Design review of the part built by this model. Coordinates are the model's own, in mm. Round coordinates to 2 decimals unless told otherwise and drop trailing zeros. Write each loop counter-clockwise with the first axis right and the second up, starting at its lowest first coordinate (ties: lowest second). Pieces come first, ordered by that corner, then holes. Notation, with made-up numbers: (47, 66) - (73, 66) arc R9 ccw to (73, 82) - close; hole circle Ø11 at (-12, 48). An arc over 180 degrees is marked (long way). Use one line per item in the form item = value.
```python
from build123d import *

# Parameters (mm, degrees)
ESQUISSE1_W                  = 19
ESQUISSE1_H                  = 3
CHANFREIN1_SIZE              = 0.2
ESQUISSE2_R                  = 0.75
ENL_V_MAT_EXTRU_1_DEPTH      = 4
ENL_V_MAT_EXTRU_1_DEPTH_BACK = 4


with BuildPart() as part:
    # Esquisse1 → Révolution1 (revolve)
    with BuildSketch(Plane.XY):
        with Locations((-5.5, 1.5)):
            Rectangle(ESQUISSE1_W, ESQUISSE1_H)
    revolve(axis=Axis((-15, 0, 0), (1, 0, 0)))

    # Chanfrein1
    chanfrein1_edges = [part.edges().sort_by_distance(p)[0] for p in [
        (-15, -3, 0),
        (4, -3, 0),
    ]]
    chamfer(chanfrein1_edges, length=CHANFREIN1_SIZE)

    # Esquisse2 → Enlèv. mat.-Extru.1 (cut, two sides)
    with BuildSketch(Plane.XY) as enl_v_mat_extru_1_sk:
        with Locations((-6.3, 0)):
            Circle(ESQUISSE2_R)
    extrude(amount=ENL_V_MAT_EXTRU_1_DEPTH, mode=Mode.SUBTRACT)
    extrude(enl_v_mat_extru_1_sk.sketch, amount=-ENL_V_MAT_EXTRU_1_DEPTH_BACK, mode=Mode.SUBTRACT)


solid = part.part
```
Q1. For P1, Ø1, axis at x = -13, z = -1.5, coming from the -Y side, flat-tipped, find the tip position at first contact; note if it passes through.
Calculated:
P1 = -2.83
Q2. We need section C-C on x = -6.3. Write out the cut boundary in (y, z).
Calculated:
outline = (-0.75, -2.9) - (-0.75, 2.9) arc R3 ccw to start; (0.75, -2.9) arc R3 ccw to (0.75, 2.9) - close
Q3. We need section B-B on x = -11.75. Write out the cut boundary in (y, z).
Calculated:
outline = circle Ø6 at (0, 0)
Q4. To check wall thickness, follow line 1 along X through (y, z) = (0, -1.7); line 2 along X through (y, z) = (-0.5, -1); line 3 along Y through (x, z) = (-6.3, -1). State the ranges of each line that lie inside material, in increasing order. Write a range as from..to.
Calculated:
line_1 = -15..-7.05, -5.55..4
line_2 = -15..-6.86, -5.74..4
line_3 = -2.83..-0.75, 0.75..2.83
Q5. We need section A-A on y = 0. Write out the cut boundary in (x, z), then the cut area to 3 significant figures.
Calculated:
outline = (-15, -2.8) - (-14.8, -3) - (-7.05, -3) - (-7.05, 3) - (-14.8, 3) - (-15, 2.8) - close; (-5.55, -3) - (3.8, -3) - (4, -2.8) - (4, 2.8) - (3.8, 3) - (-5.55, 3) - close
area = 105 mm2
